The drawing under review shows one solid part. Ordinate dimensions are in mm from its lowest x, y, z. Round coordinates to 2 decimals unless told otherwise and drop trailing zeros. Order: outer loops, then holes, each group sorted by start corner. A loop starts at its lowest first (then second) coordinate and runs counter-clockwise, first axis right, second up.
1) Consider section B-B (x = 8.89). Give the boundary of the cut face in (y, z), then the cut area to 3 significant figures.
2) To check wall thickness, follow L1, parallel to X at y = 0.8, z = 5.08; L2, parallel to Z at x = 9, y = 0.15; L3, parallel to X at y = 0.45, z = 4.5. State the ranges of each line that lie inside material, in increasing order.
3) Consider section A-A (z = 71.12). Give the boundary of the cut face in (x, y), then the cut area to 3 significant figures.
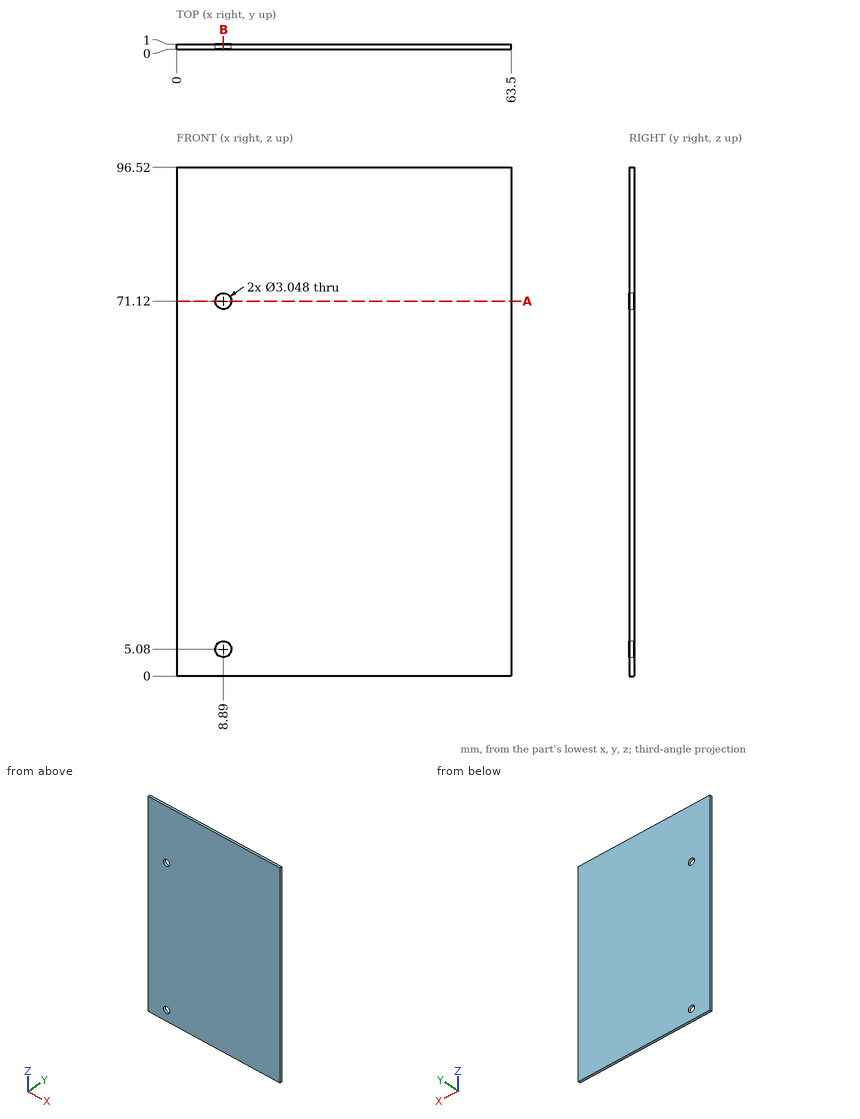
Answer below:
1. outline: (0, 0) - (1, 0) - (1, 3.56) - (0, 3.56) - close; (0, 6.6) - (1, 6.6) - (1, 69.6) - (0, 69.6) - close; (0, 72.64) - (1, 72.64) - (1, 96.52) - (0, 96.52) - close
1. area: 90.4 mm2
2. L1: x = 0 to 7.37, 10.41 to 63.5
2. L2: z = 0 to 3.56, 6.6 to 69.6, 72.64 to 96.52
2. L3: x = 0 to 7.48, 10.3 to 63.5
3. outline: (0, 0) - (7.37, 0) - (7.37, 1) - (0, 1) - close; (10.41, 0) - (63.5, 0) - (63.5, 1) - (10.41, 1) - close
3. area: 60.5 mm2
